Answer from the drawing. Dimensions are ordinates in mm from the lowest x, y and z of the part. A direction names the side the tool comes from. Give positions to 0.01 mm unless a question says otherwise; leave off trailing zeros. Write each loop counter-clockwise with the first axis right and the second up, starting at its lowest first coordinate (ties: lowest second). Pieces come first, ordered by that corner, then holes.
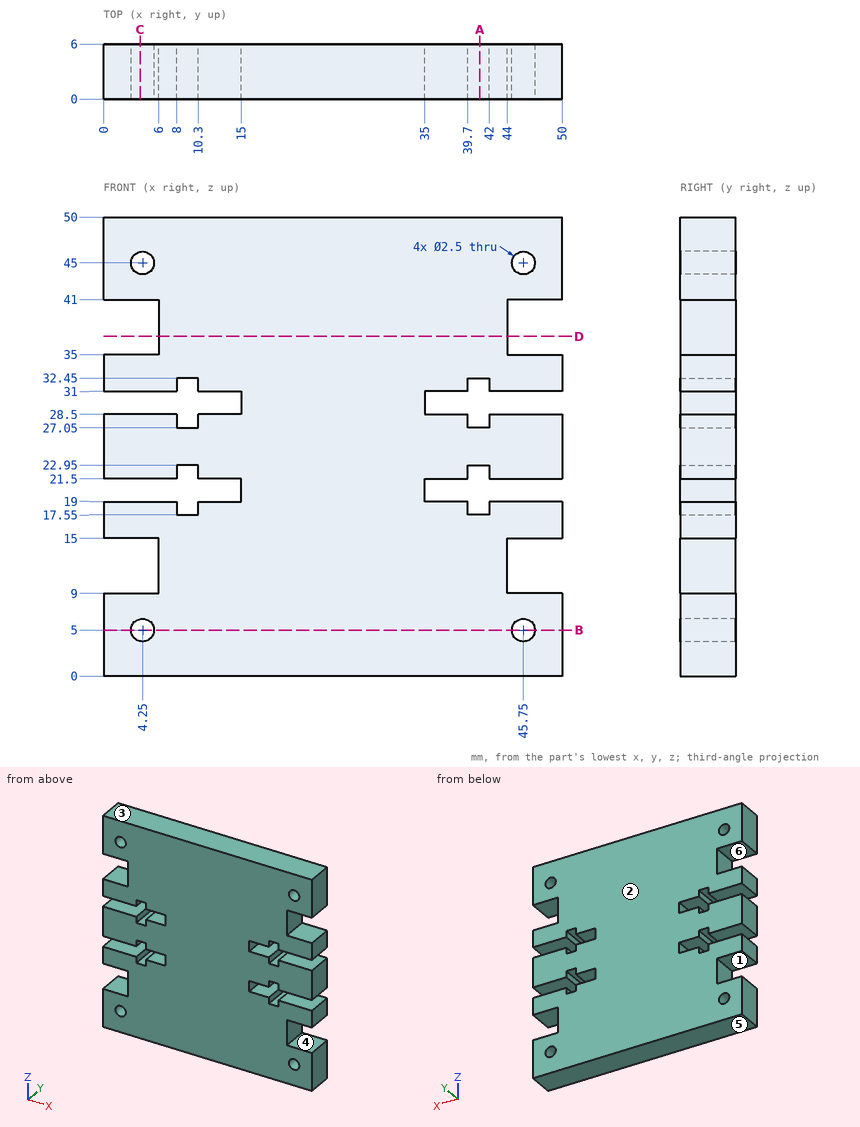
Item 1: Consider probe 1 along Z at (x, y) = (11, 4.9); probe 2 along Z at (x, y) = (41, 4.15); probe 3 along X at (y, z) = (4.4, 5.5). Determine where each line is inside the solid, lowest interval first.
Conclusion:
probe 1: z = 0 to 19, 21.5 to 28.5, 31 to 50
probe 2: z = 0 to 17.55, 22.95 to 27.05, 32.45 to 50
probe 3: x = 0 to 3.1, 5.4 to 44.6, 46.9 to 50
Item 2: Each of these flat-tipped pins is pushed along its axis until it touches: P1, Ø2, axis at x = 19.5, y = 2.5, coming from the -Z side; P2, Ø0.8, axis at y = 3.5, z = 19.5, coming from the -X side; P3, Ø2, axis at x = 4.25, z = 5, coming from the -Y side. Where does it stop, or does it pass through?
Conclusion:
P1: stops at z = 0
P2: stops at x = 15
P3: passes through
Item 3: A cutting plane is placed at B-B, the plane z = 5. Give the vertices of the cut face in (x, y), plus the area to 3 significant figures.
Conclusion:
outline: (0, 0) - (3, 0) - (3, 6) - (0, 6) - close; (5.5, 0) - (44.5, 0) - (44.5, 6) - (5.5, 6) - close; (47, 0) - (50, 0) - (50, 6) - (47, 6) - close
area: 270 mm2
Item 4: A cutting plane is placed at C-C, the plane x = 4. Give the vertices of the cut face in (y, z), plus the area to 3 significant figures.
Conclusion:
outline: (0, 0) - (6, 0) - (6, 3.78) - (0, 3.78) - close; (0, 6.22) - (6, 6.22) - (6, 9) - (0, 9) - close; (0, 15) - (6, 15) - (6, 19) - (0, 19) - close; (0, 21.5) - (6, 21.5) - (6, 28.5) - (0, 28.5) - close; (0, 31) - (6, 31) - (6, 35) - (0, 35) - close; (0, 41) - (6, 41) - (6, 43.78) - (0, 43.78) - close; (0, 46.22) - (6, 46.22) - (6, 50) - (0, 50) - close
area: 169 mm2
Item 5: A cutting plane is placed at A-A, the plane x = 41. Give the vertices of the cut face in (y, z).
Conclusion:
outline: (0, 0) - (6, 0) - (6, 17.55) - (0, 17.55) - close; (0, 22.95) - (6, 22.95) - (6, 27.05) - (0, 27.05) - close; (0, 32.45) - (6, 32.45) - (6, 50) - (0, 50) - close
Item 6: Which of the six approach directions +Z, -Z, +X, -X, +Y, -Y give full straight-line access (tool end or side, diameter ignored) to the marked faces 4, 5 and 6?
Conclusion:
face 4: +X, +Y, -Y
face 5: -Z, +X, -X, +Y, -Y
face 6: -X, +Y, -Y
Item 7: Determine the mould class of the marked faces 1, 2 and 3 for opening direction Z: pulls with the +Z half, pulls with the -Z half, needs draft (parallel to the pull), parting line crosses it, or undercut.
Conclusion:
face 1: undercut
face 2: needs draft
face 3: pulls with the +Z half
Item 8: A cutting plane is placed at D-D, the plane z = 37. Give the vertices of the cut face in (x, y).
Conclusion:
outline: (6, 0) - (44, 0) - (44, 6) - (6, 6) - close
